Read the model definition and answer for the solid it produces. Units are mm, in the model's axes. A direction names the side the tool comes from. Coordinates: 2 decimals unless noted, no trailing zeros. Order: outer loops, then holes, each group sorted by start corner. A loop starts at its lowest first (then second) coordinate and runs counter-clockwise, first axis right, second up. Notation, with made-up numbers: (42.25, -13) - (81.25, -13) arc R19 ccw to (81.25, 6) - close; hole circle Ø5 at (44.5, 12). An arc over 180 degrees is marked (long way). Write item = value, one per line.
from build123d import *

# Parameters (mm, degrees)
F1_DEPTH = 18
F2_R     = 4
F3_DEPTH = 14


with BuildPart() as f1:
    # F0 (on Front) → F1 (new body)
    with BuildSketch(Plane.XZ):
        Polygon((337.5, 194.205903), (-337.5, 194.205903), (-337.5, 169.205903), (-355.5, 169.205903), (-355.5, 119.205903), (-337.5, 119.205903), (-337.5, 69.205903), (-355.5, 69.205903), (-355.5, 19.205903), (-337.5, 19.205903), (-337.5, -30.794097), (-355.5, -30.794097), (-355.5, -80.794097), (-337.5, -80.794097), (-337.5, -130.794097), (-355.5, -130.794097), (-355.5, -180.794097), (-337.5, -180.794097), (-337.5, -205.794097), (337.5, -205.794097), (337.5, -180.794097), (355.5, -180.794097), (355.5, -130.794097), (337.5, -130.794097), (337.5, -80.794097), (355.5, -80.794097), (355.5, -30.794097), (337.5, -30.794097), (337.5, 19.205903), (355.5, 19.205903), (355.5, 69.205903), (337.5, 69.205903), (337.5, 119.205903), (355.5, 119.205903), (355.5, 169.205903), (337.5, 169.205903), align=None)
    extrude(amount=F1_DEPTH)

    # F2 (on face) → F3 (cut)
    with BuildSketch(Plane.XZ.offset(18)):
        with Locations((-155.5, -125.794097)):
            Circle(F2_R)
        with Locations((-155.5, 114.205903)):
            Circle(F2_R)
    extrude(amount=-F3_DEPTH, mode=Mode.SUBTRACT)


solid = f1.part
1) For faces 1 (the face through (-346, -9, 169.206)), 2 (the face through (337.5, -9, -106)), 3 (the face through (-337.5, -9, -5)), 4 (the face through (347, -9, 169.206)), determine the directions among +Z, -Z, +X, -X, +Y, -Y from which every point of the face is accessible in a straight line to the end or side of a thin tool.
Returned:
face_1 = +Z, -X, +Y, -Y
face_2 = +X, +Y, -Y
face_3 = -X, +Y, -Y
face_4 = +Z, +X, +Y, -Y
2) Straight lines are drawn through the part: line 1 along Z through (x, y) = (-155.5, -7.75); line 2 along X through (y, z) = (-11.5, 89). For each, find the intervals that lie inside material, in ascending order. Write a range as from..to.
Returned:
line_1 = -205.79..-129.79, -121.79..110.21, 118.21..194.21
line_2 = -337.5..337.5
3) The part is cut by section A-A (y = -8.25). Count the separate pieces of the cut face and the enclosed holes in it, and give its area (3 significant figures).
Returned:
separate_pieces = 1
enclosed_holes = 2
area = 277,000 mm^2
4) Flat-ended cylindrical pins translate along their axes: pin 1 Ø5.5 at (x, y) = (349, -12.5) entering from -Z; pin 2 Ø9 at (y, z) = (-11, 184) entering from -X; pin 3 Ø5.5 at (x, y) = (342, -8.5) entering from +Z. Find the tip coordinate at first contact, or state that the pin passes through.
Returned:
pin_1 = -180.79
pin_2 = -337.5
pin_3 = 169.21
5) The part is cut by section B-B (z = 101). Determine the outline of the cut face in (x, y), and give its area (4 significant figures).
Returned:
outline = (-337.5, -18) - (337.5, -18) - (337.5, 0) - (-337.5, 0) - close
area = 12,150 mm^2
